Verification items for the finished model (mm, model axes). A direction names the side the tool comes from. Give positions to 0.01 mm unless a question says otherwise; leave off trailing zeros. Order: outer loops, then holes, each group sorted by start corner. A loop starts at its lowest first (then second) coordinate and runs counter-clockwise, first axis right, second up. Notation, with made-up numbers: (38, 72.25) - (90, 72.25) arc R18 ccw to (90, 91.25) - close; hole circle Ø9 at (51.25, 74). An arc over 180 degrees is marked (long way). Answer as a JSON object with one key per item and string values. Group by question number.
(1) Depth check by flat-ended pin: pin 1 Ø1 at (x, z) = (-0.5, 2) entering from -Y; pin 2 Ø1 at (x, z) = (2, 3.5) entering from -Y; pin 3 Ø2 at (y, z) = (1.5, 1.5) entering from +X. Enter the tip coordinate at first touch or a pass-through.
(2) Thickness scan on line 1 (X direction, y = 1.9, z = 2.7); line 2 (Y direction, x = 1.35, z = 1.6); line 3 (X direction, y = 1.2, z = 3.65). Record the ranges inside material, lowest first.
(3) Section check A-A (z = 1.75). Record the boundary of the cut face in (x, y), then the cut area to 3 significant figures.
(4) Access from +Z, -Z, +X, -X, +Y, -Y to the whole of each face (thin tool, end or side, straight path). Record for faces 1 (the face through (-1, 0, 2)), 2 (the face through (1, 2, 2)).
(5) Section check C-C (x = 1.45). Record the boundary of the cut face in (y, z).
(6) Section check D-D (z = 1.1). Record the boundary of the cut face in (x, y).
(7) Section check B-B (y = 2.8). Record the boundary of the cut face in (x, z).
```python
from build123d import *

# Parameters (mm, degrees)
BOX008_W         = 2
BOX008_H         = 4.5
BOX008_DEPTH     = 6
EXTRUDE004_DEPTH = 6


with BuildPart() as box008:
    # Box008 → Box008 (new body)
    with BuildSketch(Plane(origin=(1, 0, -0.5), x_dir=(1, 0, 0), z_dir=(0, 0, 1))):
        with Locations((1, 2.25)):
            Rectangle(BOX008_W, BOX008_H)
    extrude(amount=BOX008_DEPTH)


with BuildPart() as obj1:
    # Sketch002 → Extrude004 (new body)
    with BuildSketch(Plane.XZ):
        Polygon((2.309699, 1.35299), (2.309699, 3.266407), (0.956709, 4.619398), (-0.956709, 4.619398), (-2.309699, 3.266407), (-2.309699, 1.35299), (-0.956709, 0), (0.956709, 0), align=None)
    extrude(amount=-EXTRUDE004_DEPTH)

    # Cut: cut Box008
    add(box008.part, mode=Mode.SUBTRACT)


solid = obj1.part
```
Solutions:
{
 "1": {"pin 1": "stops at y = 0", "pin 2": "stops at y = 4.5", "pin 3": "stops at x = 1"},
 "2": {"line 1": "x = -2.31 to 1", "line 2": "y = 4.5 to 6", "line 3": "x = -1.93 to 1"},
 "3": {"outline": "(-2.31, 0) - (1, 0) - (1, 4.5) - (2.31, 4.5) - (2.31, 6) - (-2.31, 6) - close", "area": "21.8 mm2"},
 "4": {"face 1": "+Z, -Z, +X, -X, -Y", "face 2": "+Z, -Z, +X, -Y"},
 "5": {"outline": "(4.5, 0.49) - (6, 0.49) - (6, 4.13) - (4.5, 4.13) - close"},
 "6": {"outline": "(-2.06, 0) - (1, 0) - (1, 4.5) - (2.06, 4.5) - (2.06, 6) - (-2.06, 6) - close"},
 "7": {"outline": "(-2.31, 1.35) - (-0.96, 0) - (0.96, 0) - (1, 0.04) - (1, 4.58) - (0.96, 4.62) - (-0.96, 4.62) - (-2.31, 3.27) - close"}
}
